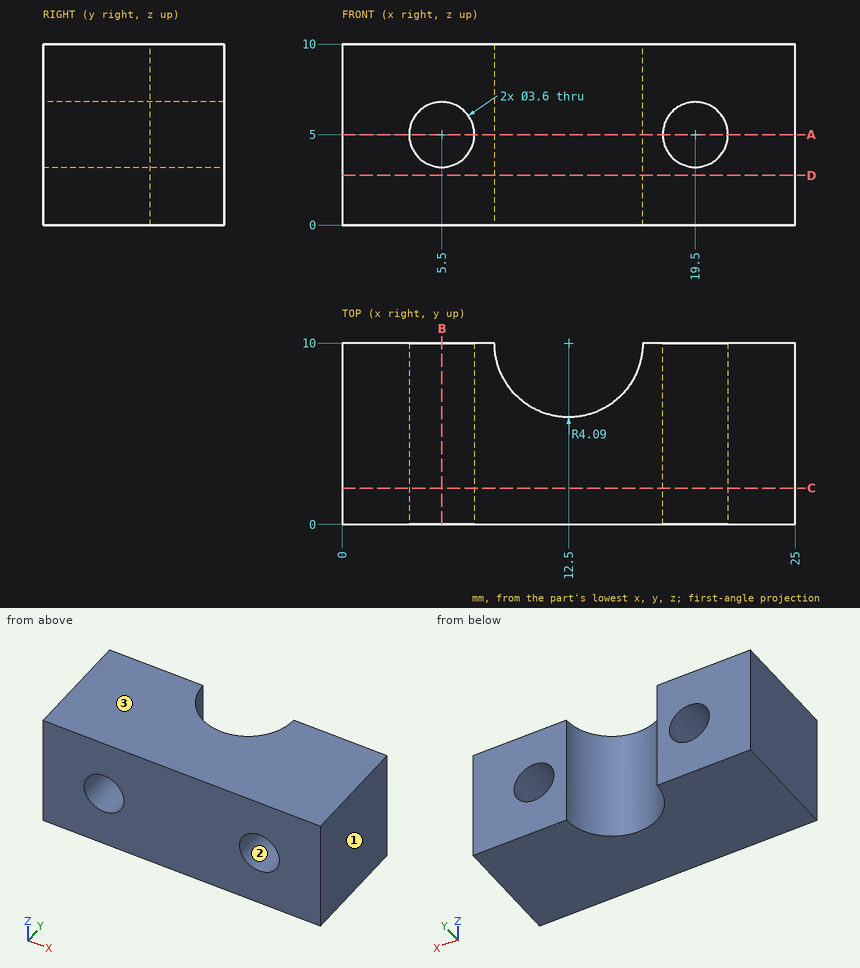
Job drawing, mm, ordinate dimensions from the low corner. One solid piece. Round coordinates to 2 decimals unless told otherwise and drop trailing zeros. Loops run counter-clockwise (first coordinate to the right, second up) from the corner with the lowest first, then second, coordinate; pieces in that order, holes last. Notation, with made-up numbers: (89.5, 51.25) -> (135.5, 51.25) arc R12 cw to (135.5, 63.25) -> close; hole circle Ø4 at (1.25, -30). An arc over 180 degrees is marked (long way). One line per item, written item: value. Start each with the question number.
Q1. Cut at B-B on x = 5.5. List the corners of the cut face in (y, z), plus the area to 3 significant figures.
Q2. Probe line 1 along X through (y, z) = (3, 5); line 2 along Z through (x, y) = (19.5, 6.5); line 3 along X through (y, z) = (7.75, 5). List the from-to ranges inside material, lowest first.
Q3. Two-plate mould, pull along Z, no slides. Class the marked faces 1, 2 and 3: released by +Z, released by -Z, zero draft, split by the parting line, or undercut.
Q4. Cut at A-A on z = 5. List the corners of the cut face in (x, y), plus the area to 3 significant figures.
Q5. Cut at C-C on y = 2. List the corners of the cut face in (x, z).
Q6. Cut at D-D on z = 2.75. List the corners of the cut face in (x, y).
Computed:
1. outline: (0, 0) -> (10, 0) -> (10, 3.2) -> (0, 3.2) -> close; (0, 6.8) -> (10, 6.8) -> (10, 10) -> (0, 10) -> close
1. area: 64.0 mm²
2. line 1: 0 to 3.7, 7.3 to 17.7, 21.3 to 25
2. line 2: 0 to 3.2, 6.8 to 10
2. line 3: 0 to 3.7, 7.3 to 9.08, 15.92 to 17.7, 21.3 to 25
3. face 1: zero draft
3. face 2: undercut
3. face 3: released by +Z
4. outline: (0, 0) -> (3.7, 0) -> (3.7, 10) -> (0, 10) -> close; (7.3, 0) -> (17.7, 0) -> (17.7, 10) -> (16.59, 10) arc R4.09 cw to (8.41, 10) -> (7.3, 10) -> close; (21.3, 0) -> (25, 0) -> (25, 10) -> (21.3, 10) -> close
4. area: 152 mm²
5. outline: (0, 0) -> (25, 0) -> (25, 10) -> (0, 10) -> close; hole circle Ø3.6 at (5.5, 5); hole circle Ø3.6 at (19.5, 5)
6. outline: (0, 0) -> (25, 0) -> (25, 10) -> (16.59, 10) arc R4.09 cw to (8.41, 10) -> (0, 10) -> close
